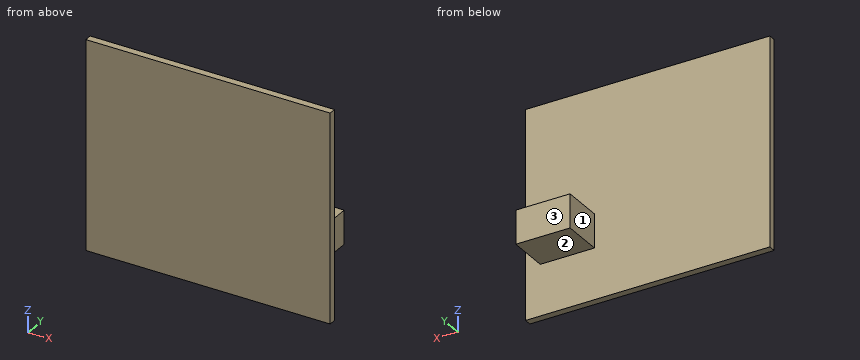
Autodesk Inventor part; units mm, degrees
ref_plane "YZ Plane" through (0, 0, 0) normal (1, 0, 0) x (0, 1, 0)
ref_plane "XZ Plane" through (0, 0, 0) normal (0, 1, 0) x (-1, 0, 0)
ref_plane "XY Plane" through (0, 0, 0) normal (0, 0, 1) x (1, 0, 0)
ref_plane "РабПлоскость1" through (475.3287, -140.8035, 12.4703) normal (0, -1, 0) x (1, 0, 0)
sketch "Эскиз1" plane through (475.3287, -140.8035, 12.4703) normal (0, -1, 0) x (1, 0, 0)
  point P0 (-475.3287, -12.4703)
sketch "Эскиз2" plane through (475.3287, -140.8035, 12.4703) normal (0, -1, 0) x (1, 0, 0)
  line L0 (-735.7265, 1024.2535) -> (1318.2521, 1024.2535)
  line L1 (1318.2521, 1024.2535) -> (1318.2521, -723.0885)
  line L2 (1318.2521, -723.0885) -> (-735.7265, -723.0885)
  line L3 (-735.7265, -723.0885) -> (-735.7265, 1024.2535)
  point P0 (-475.3287, -12.4703)
extrude "Выдавливание1" add sketch "Эскиз2" along normal blind 10
sketch "Эскиз3" plane through (475.3287, -140.8035, 12.4703) normal (0, 1, 0) x (1, 0, 0)
  line L0 (1194.1306, 12.4703) -> (738.2489, 12.4703)
  line L1 (738.2489, 12.4703) -> (738.2489, 295.0097)
  line L2 (738.2489, 295.0097) -> (1194.1306, 295.0097)
  line L3 (1194.1306, 295.0097) -> (1194.1306, 12.4703)
  point P0 (-475.3287, 12.4703)
extrude "Выдавливание2" add sketch "Эскиз3" along normal blind 390
sketch "Эскиз4" plane through (475.3287, -140.8035, 12.4703) normal (0, 1, 0) x (1, 0, 0)
  line L0 (1194.1306, 295.0097) -> (1194.1306, 12.4703)
  line L1 (1194.1306, 12.4703) -> (738.2489, 12.4703)
  line L2 (738.2489, 12.4703) -> (738.2489, 295.0097)
  line L3 (738.2489, 295.0097) -> (1194.1306, 295.0097)
  line L4 (-735.7265, 723.0885) -> (1318.2521, 723.0885)
  line L5 (-735.7265, -1024.2535) -> (-735.7265, 723.0885)
  line L6 (1318.2521, -1024.2535) -> (-735.7265, -1024.2535)
  line L7 (1318.2521, 723.0885) -> (1318.2521, -1024.2535)
  point P0 (-475.3287, 12.4703)
extrude "Выдавливание3" add sketch "Эскиз4" along normal blind 50.25
properties part number "Земля_и_Препятствия"
CAD build for the part. Positions are in the model's coordinates, mm. Face numbers are marked on the shaded views. A direction names the side the tool comes from. Round coordinates to 2 decimals unless told otherwise and drop trailing zeros. Order: outer loops, then holes, each group sorted by start corner. A loop starts at its lowest first (then second) coordinate and runs counter-clockwise, first axis right, second up. Notation, with made-up numbers: (-39, 2.5) -> (-32, 2.5) arc R28 cw to (-32, 25.5) -> close; hole circle Ø7 at (-29.5, 66). An arc over 180 degrees is marked (long way). Write item = value, one per line.
(1) Cut at C-C (y = 19.5). Write the cut outline in (x, z).
Answers follow:
outline = (1213.58, -282.54) -> (1669.46, -282.54) -> (1669.46, 0) -> (1213.58, 0) -> close
(2) Drill centre lines: L1, parallel to Y at x = 444, z = 486.5; L2, parallel to X at y = -34.5, z = -272.5; L3, parallel to Z at x = 1357, y = 102. Where is each one in solid material? Low to high.
Answers follow:
L1 = -150.8 to -90.55
L2 = 1213.58 to 1669.46
L3 = -282.54 to 0
(3) Cut at A-A (x = 1426.5). Write the cut outline in (y, z).
Answers follow:
outline = (-150.8, -710.62) -> (-90.55, -710.62) -> (-90.55, -282.54) -> (249.2, -282.54) -> (249.2, 0) -> (-90.55, 0) -> (-90.55, 1036.72) -> (-150.8, 1036.72) -> close
(4) Cut at B-B (z = 353). Write the cut outline in (x, y).
Answers follow:
outline = (-260.4, -150.8) -> (1793.58, -150.8) -> (1793.58, -90.55) -> (-260.4, -90.55) -> close
(5) Flat gauge pin, fed straight in: P1, Ø10, axis at x = 984.5, z = 242.5, coming from the +Y side. Where does the tip first touch, or does it go through?
Answers follow:
P1 = -90.55
(6) 3-axis set-ups, long thin cutter, end or side, ignore diameter. For the marked faces 1, 2 and 3: which of +Z, -Z, +X, -X, +Y, -Y reach the whole face in a straight line?
Answers follow:
face_1 = +Z, -Z, -X, +Y
face_2 = -Z, +X, -X, +Y
face_3 = +Z, -Z, +X, -X, +Y
